```python
from build123d import *

# Parameters (mm, degrees)
SKETCH1_R           = 165.1
BOSS_EXTRUDE2_DEPTH = 101.6
SKETCH2_R           = 76.2
CUT_EXTRUDE1_DEPTH  = 38.1
FILLET3_R           = 25.4
FILLET4_R           = 25.4
CUT_EXTRUDE2_START  = -38.1
SKETCH3_R           = 76.2
CUT_EXTRUDE2_DEPTH  = 38.1
FILLET5_R           = 25.4
FILLET6_R           = 25.4
SKETCH4_R           = 17.145
BOSS_EXTRUDE3_DEPTH = 38.1
BOSS_EXTRUDE4_START = 38.1
SKETCH5_R           = 17.145
BOSS_EXTRUDE4_DEPTH = 38.1
SKETCH6_R           = 9.525
CUT_EXTRUDE3_DEPTH  = 255.634208358
SKETCH7_R           = 6.35
BOSS_EXTRUDE5_DEPTH = 19.05
SKETCH8_R           = 8.89
BOSS_EXTRUDE6_DEPTH = 5.08


with BuildPart() as part:
    # Sketch1 → Boss-Extrude2 (new body)
    with BuildSketch(Plane(origin=(0, 0, 0), x_dir=(1, 0, 0), z_dir=(0, 1, 0))):
        with Locations(Location((0, 0, 0), (0, 0, 270))):
            Circle(SKETCH1_R)
    extrude(amount=BOSS_EXTRUDE2_DEPTH)

    # Sketch2 → Cut-Extrude1 (cut)
    with BuildSketch(Plane(origin=(0, 101.6, 0), x_dir=(1, 0, 0), z_dir=(0, 1, 0))):
        with Locations(Location((0, 0, 0), (0, 0, 270))):
            Circle(SKETCH2_R)
    extrude(amount=-CUT_EXTRUDE1_DEPTH, mode=Mode.SUBTRACT)

    # Fillet3
    fillet3_edges = [part.edges().sort_by_distance(p)[0] for p in [
        (0, 63.5, -76.2),
    ]]
    fillet(fillet3_edges, radius=FILLET3_R)

    # Fillet4
    fillet4_edges = [part.edges().sort_by_distance(p)[0] for p in [
        (0, 101.6, -165.1),
    ]]
    fillet(fillet4_edges, radius=FILLET4_R)

    # Sketch3 → Cut-Extrude2 (cut)
    with BuildSketch(Plane(origin=(0, 0, 0), x_dir=(-1, 0, 0), z_dir=(0, -1, 0)).offset(CUT_EXTRUDE2_START)):
        with Locations(Location((0, 0, 0), (0, 0, 270))):
            Circle(SKETCH3_R)
    extrude(amount=CUT_EXTRUDE2_DEPTH, mode=Mode.SUBTRACT)

    # Fillet5
    fillet5_edges = [part.edges().sort_by_distance(p)[0] for p in [
        (0, 38.1, -76.2),
    ]]
    fillet(fillet5_edges, radius=FILLET5_R)

    # Fillet6
    fillet6_edges = [part.edges().sort_by_distance(p)[0] for p in [
        (0, 0, -165.1),
    ]]
    fillet(fillet6_edges, radius=FILLET6_R)

    # Sketch4 → Boss-Extrude3 (add)
    with BuildSketch(Plane(origin=(0, 38.1, 0), x_dir=(-1, 0, 0), z_dir=(0, -1, 0))):
        with Locations(Location((0, 0, 0), (0, 0, 270))):
            Circle(SKETCH4_R)
    extrude(amount=BOSS_EXTRUDE3_DEPTH)

    # Sketch5 → Boss-Extrude4 (add)
    with BuildSketch(Plane(origin=(0, 63.5, 0), x_dir=(1, 0, 0), z_dir=(0, 1, 0)).offset(BOSS_EXTRUDE4_START)):
        with Locations(Location((0, 0, 0), (0, 0, 270))):
            Circle(SKETCH5_R)
    extrude(amount=-BOSS_EXTRUDE4_DEPTH)

    # Sketch6 → Cut-Extrude3 (cut, through all)
    with BuildSketch(Plane(origin=(0, 101.6, 0), x_dir=(1, 0, 0), z_dir=(0, 1, 0))):
        with Locations(Location((0, 0, 0), (0, 0, 270))):
            Circle(SKETCH6_R)
    extrude(amount=-CUT_EXTRUDE3_DEPTH, mode=Mode.SUBTRACT)

    # Sketch7 → Boss-Extrude5 (add)
    with BuildSketch(Plane(origin=(0, 63.5, 0), x_dir=(1, 0, 0), z_dir=(0, 1, 0))):
        with Locations(Location((-37.785648207, -13.547919649, 0), (0, 0, 90))):
            Circle(SKETCH7_R)
    extrude(amount=BOSS_EXTRUDE5_DEPTH)

    # Sketch8 → Boss-Extrude6 (add)
    with BuildSketch(Plane(origin=(0, 82.55, 0), x_dir=(1, 0, 0), z_dir=(0, 1, 0))):
        with Locations(Location((-37.785648207, -13.547919649, 0), (0, 0, 270))):
            Circle(SKETCH8_R)
    extrude(amount=BOSS_EXTRUDE6_DEPTH)


solid = part.part
```
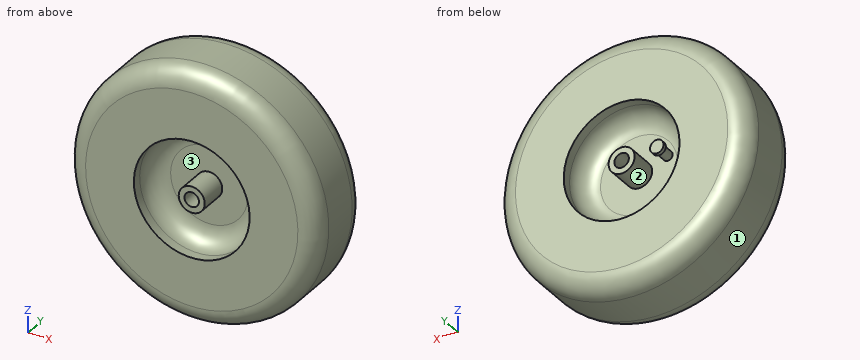
For this review, take the finished solid that the model builds, in its own axes (mm). Face numbers are marked on the shaded views. A direction names the side the tool comes from. Round coordinates to 2 decimals unless told otherwise and drop trailing zeros. Loops run counter-clockwise (first coordinate to the right, second up) from the corner with the lowest first, then second, coordinate; pieces in that order, holes last.
Q1. Add section C-C on y = 44.5. Write out the cut boundary in (x, z) (3 decimals), plus the area to 3 significant figures.
Result sheet:
outline: circle Ø330.2 at (0, 0); hole circle Ø19.05 at (0, 0)
area: 85,300 mm2
Q2. Insertion check: pin 1 Ø8 at (y, z) = (15, -58) entering from +X; pin 2 Ø6 at (x, y) = (-58, 74) entering from +Z; pin 3 Ø1 at (x, y) = (124.5, 25) entering from -Z. Each pin has a flat end and moves straight along its axis. Give the tip position at first contact, or say it passes through.
Result sheet:
pin 1: stops at x = 154.38
pin 2: stops at z = 155.67
pin 3: stops at z = -109
Q3. Machinability: for the marked faces 1, 2 and 3, which of the approach directions +Z, -Z, +X, -X, +Y, -Y give a long, thin tool a straight path to every point of the face, cutting with its end or side? Answer none if there is none.
Result sheet:
face 1: +Y, -Y
face 2: +Y
face 3: -Y
Q4. To check wall thickness, follow line 1 along X through (y, z) = (92, 0) (3 decimals); line 2 along X through (y, z) = (76, 0) (3 decimals); line 3 along X through (y, z) = (17.5, 38). State the ranges of each line that lie inside material, in increasing order.
Result sheet:
line 1: x = -159.588 to -76.2, -17.145 to -9.525, 9.525 to 17.145, 76.2 to 159.588
line 2: x = -165.1 to -72.68, -17.145 to -9.525, 9.525 to 17.145, 72.68 to 165.1
line 3: x = -159.37 to -65.52, 65.52 to 159.37
